```python
from build123d import *

# Parameters (mm, degrees)
SKETCH1_R                = 12.7
BOSS_EXTRUDE1_DEPTH      = 12.7
BOSS_EXTRUDE1_DEPTH_BACK = 12.7
FILLET1_R                = 76.2


with BuildPart() as part:
    # Sketch1 → Boss-Extrude1 (new body, two sides)
    with BuildSketch(Plane.XY) as boss_extrude1_sk:
        with BuildLine():
            ThreePointArc((-381, -304.8), (-377.280256121, -313.780256121), (-368.3, -317.5))
            Line((-368.3, -317.5), (482.162068966, -317.5))
            Line((482.162068966, -317.5), (241.3, 0))
            Line((241.3, 0), (190.5, 0))
            ThreePointArc((190.5, 0), (0, -190.5), (-190.5, 0))
            Line((-190.5, 0), (-241.3, 0))
            Line((-241.3, 0), (-381, -184.15))
            Line((-381, -184.15), (-381, -304.8))
        make_face()
        with Locations((208.543385896, -55.879031838)):
            Circle(SKETCH1_R, mode=Mode.SUBTRACT)
        with Locations((-55.879031838, -208.543385896)):
            Circle(SKETCH1_R, mode=Mode.SUBTRACT)
        with Locations((-208.543385896, -55.879031838)):
            Circle(SKETCH1_R, mode=Mode.SUBTRACT)
        with Locations((-152.664354058, -152.664354058)):
            Circle(SKETCH1_R, mode=Mode.SUBTRACT)
        with Locations((55.879031838, -208.543385896)):
            Circle(SKETCH1_R, mode=Mode.SUBTRACT)
        with Locations((152.664354058, -152.664354058)):
            Circle(SKETCH1_R, mode=Mode.SUBTRACT)
    extrude(amount=BOSS_EXTRUDE1_DEPTH)
    extrude(boss_extrude1_sk.sketch, amount=-BOSS_EXTRUDE1_DEPTH_BACK)

    # Fillet1
    fillet1_edges = [part.edges().sort_by_distance(p)[0] for p in [
        (-241.3, 0, 0),
        (241.3, 0, 0),
    ]]
    fillet(fillet1_edges, radius=FILLET1_R)


solid = part.part
```
Model file for the job. Use its own axes, mm. Give positions to 0.01 mm unless a question says otherwise; leave off trailing zeros. Loops run counter-clockwise (first coordinate to the right, second up) from the corner with the lowest first, then second, coordinate; pieces in that order, holes last. Notation, with made-up numbers: (39.25, -32) -> (82.25, -32) arc R8 cw to (82.25, -20) -> close; hole circle Ø4 at (16, 39.25). An arc over 180 degrees is marked (long way). Write each question's results on one line, items separated by ' | '.
(1) Pull direction X, two halves, no side cores. Call faces 1 (the cylindrical face through (4.189, -190.454, 0.178)), 2 (the cylindrical face through (236.911, -7.734, 0.178)), 3 (the flat face through (-381, -244, 0)), 4 (the flat face through (45, -192, -12.7)): released by +X, released by -X, zero draft, split by the parting line, or undercut.
Geometry results:
face 1: undercut | face 2: released by +X | face 3: released by -X | face 4: zero draft
(2) Cut at B-B on x = -154.5. List the corners of the cut face in (y, z).
Geometry results:
outline: (-317.5, -12.7) -> (-165.23, -12.7) -> (-165.23, 12.7) -> (-317.5, 12.7) -> close; (-140.1, -12.7) -> (-111.45, -12.7) -> (-111.45, 12.7) -> (-140.1, 12.7) -> close
(3) Cut at D-D on x = 0. List the corners of the cut face in (y, z), and give its area (3 significant figures).
Geometry results:
outline: (-317.5, -12.7) -> (-190.5, -12.7) -> (-190.5, 12.7) -> (-317.5, 12.7) -> close | area: 3,230 mm²
(4) Cut at C-C on z = -7.75. List the corners of the cut face in (x, y).
Geometry results:
outline: (-381, -304.8) arc R12.7 ccw to (-368.3, -317.5) -> (482.16, -317.5) -> (264.17, -30.15) arc R76.2 ccw to (203.46, 0) -> (190.5, 0) arc R190.5 cw to (-190.5, 0) -> (-203.46, 0) arc R76.2 ccw to (-264.17, -30.15) -> (-381, -184.15) -> close; hole circle Ø25.4 at (-208.54, -55.88); hole circle Ø25.4 at (-152.66, -152.66); hole circle Ø25.4 at (-55.88, -208.54); hole circle Ø25.4 at (55.88, -208.54); hole circle Ø25.4 at (152.66, -152.66); hole circle Ø25.4 at (208.54, -55.88)
(5) Cut at A-A on y = -76. List the corners of the cut face in (x, z).
Geometry results:
outline: (-298.96, -12.7) -> (-174.68, -12.7) -> (-174.68, 12.7) -> (-298.96, 12.7) -> close; (174.68, -12.7) -> (298.96, -12.7) -> (298.96, 12.7) -> (174.68, 12.7) -> close
(6) Flat gauge pin, fed straight in: pin 1 Ø8 at (y, z) = (-93, 0) entering from -X. Where does the tip first touch, or does it go through?
Geometry results:
pin 1: stops at x = -314.89
(7) Probe line 1 along X through (y, z) = (-160, -10); line 2 along X through (y, z) = (-58.5, -2.75); line 3 along X through (y, z) = (-126.5, -10). List the from-to ranges inside material, lowest first.
Geometry results:
line 1: x = -362.68 to -163.03, -142.3 to -103.39, 103.39 to 142.3, 163.03 to 362.68 | line 2: x = -285.68 to -220.97, -196.12 to -181.3, 181.3 to 196.12, 220.97 to 285.68 | line 3: x = -337.27 to -142.44, 142.44 to 337.27
